Geometry: see drawing. Coordinates: mm, zero at the bounding-box minimum. Round coordinates to 2 decimals unless told otherwise and drop trailing zeros. Write each loop counter-clockwise with the first axis right and the second up, starting at its lowest first coordinate (ties: lowest second). Pieces come first, ordered by that corner, then holes.
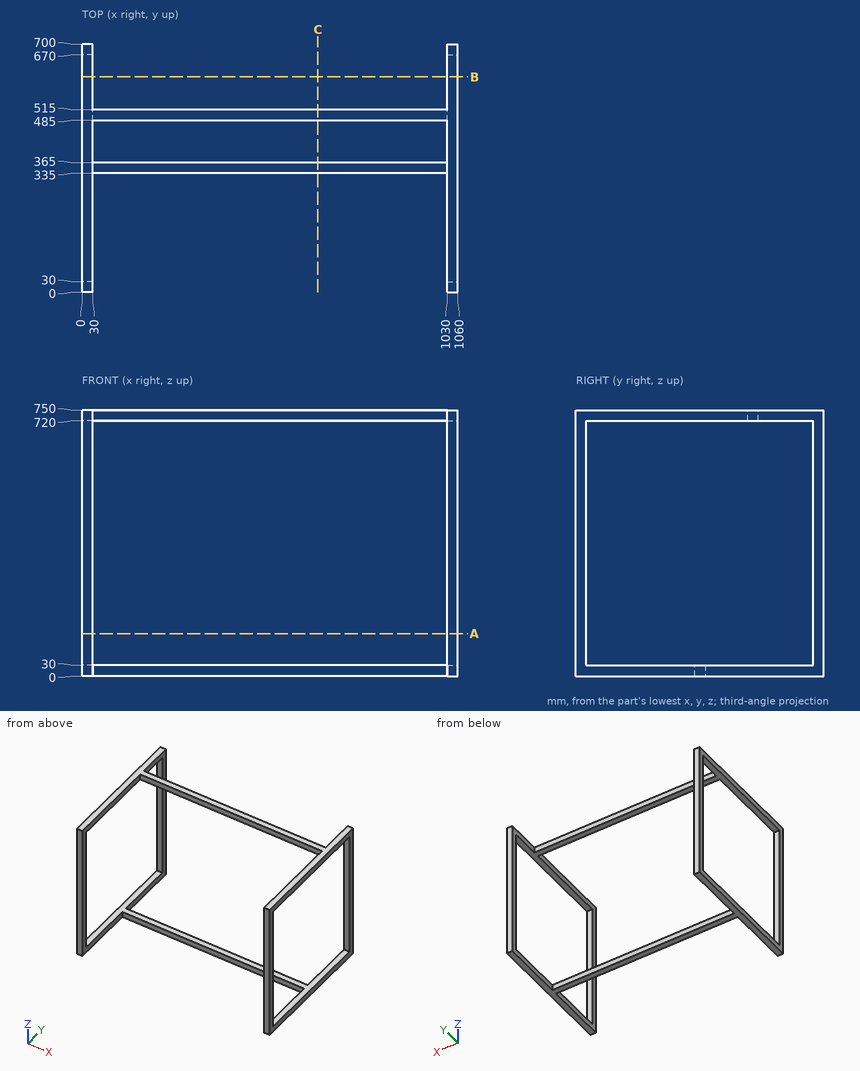
1) Section query B-B on y = 607.5. Return the cut outline in (x, z), then the cut area to 3 significant figures.
Taken from the geometry:
outline: (0, 0) - (30, 0) - (30, 30) - (0, 30) - close; (0, 720) - (30, 720) - (30, 750) - (0, 750) - close; (1030, 0) - (1060, 0) - (1060, 30) - (1030, 30) - close; (1030, 720) - (1060, 720) - (1060, 750) - (1030, 750) - close
area: 3,600 mm2
2) Section query A-A on z = 119.5. Return the cut outline in (x, y), then the cut area to 3 significant figures.
Taken from the geometry:
outline: (0, 0) - (30, 0) - (30, 30) - (0, 30) - close; (0, 670) - (30, 670) - (30, 700) - (0, 700) - close; (1030, 0) - (1060, 0) - (1060, 30) - (1030, 30) - close; (1030, 670) - (1060, 670) - (1060, 700) - (1030, 700) - close
area: 3,600 mm2
3) Contact query for flat-ended pins moving along their axis: P1, Ø9, axis at x = 779.5, z = 8.5, coming from the +Y side; P2, Ø24, axis at x = 13.5, z = 440.5, coming from the -Y side; P3, Ø24, axis at x = 642.5, z = 15.5, coming from the -Y side. Output: stop coordinate, or through.
Taken from the geometry:
P1: stops at y = 365
P2: stops at y = 0
P3: stops at y = 335
4) Section query C-C on x = 665. Return the cut outline in (y, z).
Taken from the geometry:
outline: (335, 0) - (365, 0) - (365, 30) - (335, 30) - close; (485, 720) - (515, 720) - (515, 750) - (485, 750) - close
5) Material intervals for line 1 (Z direction, x = 566, y = 353); line 2 (Z direction, x = 133.5, y = 497), sorted ascending.
Taken from the geometry:
line 1: z = 0 to 30
line 2: z = 720 to 750
